Design review of the part built by this model. Coordinates are the model's own, in mm. A direction names the side the tool comes from. Coordinates: 2 decimals unless noted, no trailing zeros. Answer in a Markdown table with one row per item.
from build123d import *

# Parameters (mm, degrees)
BOSS_EXTRUDE1_DEPTH  = 8
SKETCH2_R            = 37.5
BOSS_EXTRUDE2_DEPTH  = 2
FILLET1_R            = 1.5
FILLET1_OF_MIRROR1_R = 1.5
SKETCH3_R            = 1.6
CUT_EXTRUDE1_DEPTH   = 38.5000001
CUT_EXTRUDE2_START   = -10
SKETCH3_3_R          = 1.6
CUT_EXTRUDE2_DEPTH   = 4.1
SKETCH4_W            = 5.5
SKETCH4_H            = 4.1
CUT_EXTRUDE3_DEPTH   = 10
CUT_EXTRUDE4_START   = -5
SKETCH5_R            = 2.9
CUT_EXTRUDE4_DEPTH   = 19.4000001


with BuildPart() as part:
    # Sketch1 → Boss-Extrude1 (new body, symmetric)
    with BuildSketch(Plane(origin=(0, 0, 0), x_dir=(1, 0, 0), z_dir=(0, 1, 0))):
        with BuildLine():
            ThreePointArc((3.096965553, 34.902871005), (0, 31.94), (-3.096965553, 34.902871005))
            ThreePointArc((-3.096965553, 34.902871005), (-3.923235243, 34.819675835), (-4.747301293, 34.716922825))
            ThreePointArc((-4.747301293, 34.716922825), (-7.107318631, 31.139197515), (-10.785937615, 33.33864349))
            ThreePointArc((-10.785937615, 33.33864349), (-11.572978331, 33.073671894), (-12.353518629, 32.79012317))
            ThreePointArc((-12.353518629, 32.79012317), (-13.858246627, 28.776945641), (-17.934057726, 30.102677181))
            ThreePointArc((-17.934057726, 30.102677181), (-18.642403961, 29.669215941), (-19.340278957, 29.219089819))
            ThreePointArc((-19.340278957, 29.219089819), (-19.914264271, 24.97169755), (-24.182889297, 25.357236941))
            ThreePointArc((-24.182889297, 25.357236941), (-24.777021613, 24.777021613), (-25.357236941, 24.182889297))
            ThreePointArc((-25.357236941, 24.182889297), (-24.97169755, 19.914264271), (-29.219089819, 19.340278957))
            ThreePointArc((-29.219089819, 19.340278957), (-29.669215941, 18.642403961), (-30.102677181, 17.934057726))
            ThreePointArc((-30.102677181, 17.934057726), (-28.776945641, 13.858246627), (-32.79012317, 12.353518629))
            ThreePointArc((-32.79012317, 12.353518629), (-33.073671894, 11.572978331), (-33.33864349, 10.785937615))
            ThreePointArc((-33.33864349, 10.785937615), (-31.139197515, 7.107318631), (-34.716922825, 4.747301293))
            ThreePointArc((-34.716922825, 4.747301293), (-34.819675835, 3.923235243), (-34.902871005, 3.096965553))
            ThreePointArc((-34.902871005, 3.096965553), (-31.94, 0), (-34.902871005, -3.096965553))
            ThreePointArc((-34.902871005, -3.096965553), (-34.819675835, -3.923235243), (-34.716922825, -4.747301293))
            ThreePointArc((-34.716922825, -4.747301293), (-31.139197515, -7.107318631), (-33.33864349, -10.785937615))
            ThreePointArc((-33.33864349, -10.785937615), (-33.073671894, -11.572978331), (-32.79012317, -12.353518629))
            ThreePointArc((-32.79012317, -12.353518629), (-28.776945641, -13.858246627), (-30.102677181, -17.934057726))
            ThreePointArc((-30.102677181, -17.934057726), (-29.669215941, -18.642403961), (-29.219089819, -19.340278957))
            ThreePointArc((-29.219089819, -19.340278957), (-24.97169755, -19.914264271), (-25.357236941, -24.182889297))
            ThreePointArc((-25.357236941, -24.182889297), (-24.777021613, -24.777021613), (-24.182889297, -25.357236941))
            ThreePointArc((-24.182889297, -25.357236941), (-19.914264271, -24.97169755), (-19.340278957, -29.219089819))
            ThreePointArc((-19.340278957, -29.219089819), (-18.642403961, -29.669215941), (-17.934057726, -30.102677181))
            ThreePointArc((-17.934057726, -30.102677181), (-13.858246627, -28.776945641), (-12.353518629, -32.79012317))
            ThreePointArc((-12.353518629, -32.79012317), (-11.572978331, -33.073671894), (-10.785937615, -33.33864349))
            ThreePointArc((-10.785937615, -33.33864349), (-7.107318631, -31.139197515), (-4.747301293, -34.716922825))
            ThreePointArc((-4.747301293, -34.716922825), (-3.923235243, -34.819675835), (-3.096965553, -34.902871005))
            ThreePointArc((-3.096965553, -34.902871005), (0, -31.94), (3.096965553, -34.902871005))
            ThreePointArc((3.096965553, -34.902871005), (3.923235243, -34.819675835), (4.747301293, -34.716922825))
            ThreePointArc((4.747301293, -34.716922825), (7.107318631, -31.139197515), (10.785937615, -33.33864349))
            ThreePointArc((10.785937615, -33.33864349), (11.572978331, -33.073671894), (12.353518629, -32.79012317))
            ThreePointArc((12.353518629, -32.79012317), (13.858246627, -28.776945641), (17.934057726, -30.102677181))
            ThreePointArc((17.934057726, -30.102677181), (18.642403961, -29.669215941), (19.340278957, -29.219089819))
            ThreePointArc((19.340278957, -29.219089819), (19.914264271, -24.97169755), (24.182889297, -25.357236941))
            ThreePointArc((24.182889297, -25.357236941), (24.777021613, -24.777021613), (25.357236941, -24.182889297))
            ThreePointArc((25.357236941, -24.182889297), (24.97169755, -19.914264271), (29.219089819, -19.340278957))
            ThreePointArc((29.219089819, -19.340278957), (29.669215941, -18.642403961), (30.102677181, -17.934057726))
            ThreePointArc((30.102677181, -17.934057726), (28.776945641, -13.858246627), (32.79012317, -12.353518629))
            ThreePointArc((32.79012317, -12.353518629), (33.073671894, -11.572978331), (33.33864349, -10.785937615))
            ThreePointArc((33.33864349, -10.785937615), (31.139197515, -7.107318631), (34.716922825, -4.747301293))
            ThreePointArc((34.716922825, -4.747301293), (34.819675835, -3.923235243), (34.902871005, -3.096965553))
            ThreePointArc((34.902871005, -3.096965553), (31.94, 0), (34.902871005, 3.096965553))
            ThreePointArc((34.902871005, 3.096965553), (34.819675835, 3.923235243), (34.716922825, 4.747301293))
            ThreePointArc((34.716922825, 4.747301293), (31.139197515, 7.107318631), (33.33864349, 10.785937615))
            ThreePointArc((33.33864349, 10.785937615), (33.073671894, 11.572978331), (32.79012317, 12.353518629))
            ThreePointArc((32.79012317, 12.353518629), (28.776945641, 13.858246627), (30.102677181, 17.934057726))
            ThreePointArc((30.102677181, 17.934057726), (29.669215941, 18.642403961), (29.219089819, 19.340278957))
            ThreePointArc((29.219089819, 19.340278957), (24.97169755, 19.914264271), (25.357236941, 24.182889297))
            ThreePointArc((25.357236941, 24.182889297), (24.777021613, 24.777021613), (24.182889297, 25.357236941))
            ThreePointArc((24.182889297, 25.357236941), (19.914264271, 24.97169755), (19.340278957, 29.219089819))
            ThreePointArc((19.340278957, 29.219089819), (18.642403961, 29.669215941), (17.934057726, 30.102677181))
            ThreePointArc((17.934057726, 30.102677181), (13.858246627, 28.776945641), (12.353518629, 32.79012317))
            ThreePointArc((12.353518629, 32.79012317), (11.572978331, 33.073671894), (10.785937615, 33.33864349))
            ThreePointArc((10.785937615, 33.33864349), (7.107318631, 31.139197515), (4.747301293, 34.716922825))
            ThreePointArc((4.747301293, 34.716922825), (3.923235243, 34.819675835), (3.096965553, 34.902871005))
        make_face()
        with BuildLine():
            ThreePointArc((1.658312395, 2.5), (0, -3), (-1.658312395, 2.5))
            Line((-1.658312395, 2.5), (1.658312395, 2.5))
        make_face(mode=Mode.SUBTRACT)
    extrude(amount=BOSS_EXTRUDE1_DEPTH, both=True)

    # Sketch2 → Boss-Extrude2 (add)
    with BuildSketch(Plane(origin=(0, 8, 0), x_dir=(1, 0, 0), z_dir=(0, 1, 0))):
        Circle(SKETCH2_R)
        with BuildLine():
            Line((-1.658312395, 2.5), (1.658312395, 2.5))
            ThreePointArc((1.658312395, 2.5), (0, -3), (-1.658312395, 2.5))
        make_face(mode=Mode.SUBTRACT)
    boss_extrude2 = extrude(amount=BOSS_EXTRUDE2_DEPTH)

    # Fillet1
    fillet1_edges = [part.edges().sort_by_distance(p)[0] for p in [
        (-37.5, 8, 0),
    ]]
    fillet(fillet1_edges, radius=FILLET1_R)

    # Mirror1: Boss-Extrude2 across plane
    add(boss_extrude2.mirror(Plane.ZX))

    # Fillet1 of Mirror1
    fillet1_of_mirror1_edges = [part.edges().sort_by_distance(p)[0] for p in [
        (-37.5, -8, 0),
    ]]
    fillet(fillet1_of_mirror1_edges, radius=FILLET1_OF_MIRROR1_R)

    # Sketch3 → Cut-Extrude1 (cut, through all)
    with BuildSketch(Plane.XY):
        Circle(SKETCH3_R)
    extrude(amount=-CUT_EXTRUDE1_DEPTH, mode=Mode.SUBTRACT)

    # Sketch3_3 → Cut-Extrude2 (cut)
    with BuildSketch(Plane.XY.offset(CUT_EXTRUDE2_START)):
        Polygon((0, -3.175426481), (2.75, -1.58771324), (2.75, 1.58771324), (0, 3.175426481), (-2.75, 1.58771324), (-2.75, -1.58771324), align=None)
        Circle(SKETCH3_3_R, mode=Mode.SUBTRACT)
    extrude(amount=-CUT_EXTRUDE2_DEPTH, mode=Mode.SUBTRACT)

    # Sketch4 → Cut-Extrude3 (cut)
    with BuildSketch(Plane(origin=(0, -10, 0), x_dir=(-1, 0, 0), z_dir=(0, -1, 0))):
        with Locations((0, 12.05)):
            Rectangle(SKETCH4_W, SKETCH4_H)
    extrude(amount=-CUT_EXTRUDE3_DEPTH, mode=Mode.SUBTRACT)

    # Sketch5 → Cut-Extrude4 (cut, through all)
    with BuildSketch(Plane.XY.offset(-14.1).offset(CUT_EXTRUDE4_START)):
        Circle(SKETCH5_R)
    extrude(amount=-CUT_EXTRUDE4_DEPTH, mode=Mode.SUBTRACT)


solid = part.part
(1) Add section A-A, the plane y = -6. Give the number of separate pieces and of enclosed holes in the cut face, and give its area (3 significant figures).
Return value:
| item | result |
|---|---|
| separate pieces | 1 |
| enclosed holes | 2 |
| area | 3,390 mm2 |
(2) For line 1 along X through (y, z) = (0, -15.35); line 2 along Y through (x, z) = (0, -18.05); line 3 along X through (y, z) = (0, -29.75), list the stretches that pass through material, from the lowest coordinate up. Write a range as from..to.
Return value:
| item | result |
|---|---|
| line 1 | x = -28.47..-1.6, 1.6..28.47 |
| line 2 | y = -10..-1.6, 1.6..10 |
| line 3 | x = -18.51..-17.71, -12.69..-2.9, 2.9..12.69, 17.71..18.51 |
(3) For faces 1 (the cylindrical face through (-3.93, 0.11, 34.82)), 2 (the cylindrical face through (19.97, 0.11, -24.93)), 3 (the flat face through (-1.36, 2.39, -12.02)), 4 (the flat face through (1.25, -1.25, -19.1)), list the 3-axis set-ups (+Z, -Z, +X, -X, +Y, -Y) from which the entire face can be reached by the end or side of a thin tool; tool diameter is ignored.
Return value:
| item | result |
|---|---|
| face 1 | +Z, -X |
| face 2 | none |
| face 3 | -Y |
| face 4 | -Z |
(4) Insertion check: pin 1 Ø3 at (x, y) = (22.5, 7.5) entering from +Z; pin 2 Ø3 at (x, y) = (0, 0) entering from -Z; pin 3 Ø3.5 at (x, y) = (0, 0) entering from -Z. Each pin has a flat end and moves straight along its axis. Give the tip position at first contact, or say it passes through.
Return value:
| item | result |
|---|---|
| pin 1 | stops at z = 30.38 |
| pin 2 | stops at z = 2.6 |
| pin 3 | stops at z = -19.1 |
(5) Draft analysis for pull direction Z (two halves, no side actions). For faces 5 (the flat face through (8, -10, -1)), 6 (the cylindrical face through (-25.014, 0.112, 19.863)), 7 (the cylindrical face through (-4.88, -9.75, -37.18)), 8 (the cylindrical face through (3.93, 0.11, -34.82)), state which applies: pulls with the +Z half, pulls with the -Z half, needs draft (parallel to the pull), parting line crosses it, or undercut.
Return value:
| item | result |
|---|---|
| face 5 | needs draft |
| face 6 | undercut |
| face 7 | parting line crosses it |
| face 8 | pulls with the -Z half |
